```python
from build123d import *

# Parameters (mm, degrees)
F1_DEPTH     = 2.37
F3_DEPTH     = 2.37
F5_DEPTH     = 2.25
F6_DEPTH     = 0.75
F7_SIZE      = 0.5
F8_T4_ANGLE  = 81.836383008
F8_T10_ANGLE = 99.1168662244
F10_DEPTH    = 3.12


# Not quite as in the source:
# - a fillet or chamfer that OpenCascade refuses, or shapes differently, is made with other operations: its cross-section is extruded or revolved along the edge and cut away or added


with BuildPart() as f1:
    # F0 (on Right) → F1 (new body)
    with BuildSketch(Plane.YZ):
        with BuildLine():
            ThreePointArc((-46.5614527995, 89.8296507657), (-59.272592692, 87.6283434753), (-70.5032497848, 81.2808106933))
            Line((-70.5032497848, 81.2808106933), (-46.5614527995, 52.0296507657))
            Line((-46.5614527995, 52.0296507657), (-42.2863249385, 46.8064651858))
            ThreePointArc((-42.2863249385, 46.8064651858), (-37.3697308445, 54.2738686288), (-37.5751261635, 63.2121472344))
            Line((-37.5751261635, 63.2121472344), (-46.5614527995, 89.8296507657))
        make_face()
        with BuildLine():
            Line((-46.5614527995, 52.0296507657), (-70.5032497848, 81.2808106933))
            ThreePointArc((-70.5032497848, 81.2808106933), (-78.9453750126, 71.5263577209), (-83.6157032002, 59.501098232))
            Line((-83.6157032002, 59.501098232), (-59.2995451707, 45.4309163095))
            ThreePointArc((-59.2995451707, 45.4309163095), (-50.5782061954, 43.4628568222), (-42.2863249385, 46.8064651858))
            Line((-42.2863249385, 46.8064651858), (-46.5614527995, 52.0296507657))
        make_face()
    extrude(amount=F1_DEPTH)

    # F2 (on face) → F3 (join)
    with BuildSketch(Plane(origin=(0, 0, 0), x_dir=(0, -1, 0), z_dir=(-1, 0, 0))):
        with BuildLine():
            ThreePointArc((84.0721339402, 59.7652050675), (70.8199402211, 81.6677307982), (46.7301322311, 90.3292793181))
            Line((46.7301322311, 90.3292793181), (46.5614527995, 89.8296507657))
            ThreePointArc((46.5614527995, 89.8296507657), (70.5032497848, 81.2808106933), (83.6157032002, 59.501098232))
            Line((83.6157032002, 59.501098232), (84.0721339402, 59.7652050675))
        make_face()
        with BuildLine():
            ThreePointArc((84.9830454985, 60.2922904452), (71.4533210937, 82.4415710079), (47.0667704776, 91.3264019551))
            Line((47.0667704776, 91.3264019551), (46.7301322311, 90.3292793181))
            ThreePointArc((46.7301322311, 90.3292793181), (70.8199402211, 81.6677307982), (84.0721339402, 59.7652050675))
            Line((84.0721339402, 59.7652050675), (84.9830454985, 60.2922904452))
        make_face()
    extrude(amount=-F3_DEPTH)

    # F4 (on face) → F5 (cut)
    with BuildSketch(Plane.YZ.offset(2.37)):
        with BuildLine():
            ThreePointArc((-73.802497152, 53.8228330154), (-63.8527506222, 73.1554884912), (-42.9348652938, 79.0876969454))
            Line((-42.9348652938, 79.0876969454), (-46.7301322311, 90.3292793181))
            ThreePointArc((-46.7301322311, 90.3292793181), (-70.8199402211, 81.6677307982), (-84.0721339402, 59.7652050675))
            Line((-84.0721339402, 59.7652050675), (-73.802497152, 53.8228330154))
        make_face()
    extrude(amount=-F5_DEPTH, mode=Mode.SUBTRACT)

    # F6 (add): a face of the model
    f6_faces = [f1.faces().sort_by_distance(p)[0] for p in [
        (0, -58.3598378742, 66.4444605195),
    ]]
    extrude(f6_faces, amount=F6_DEPTH)

    # F7
    f7_edges = [f1.edges().sort_by_distance(p)[0] for p in [
        (2.37, -71.453321, 82.441571),
        (2.37, -63.852751, 73.155488),
    ]]
    chamfer(f7_edges, length=F7_SIZE)

    # F8: fillet of radius 0.5 on 2 edges, made by hand


with BuildPart() as f8_tool2:
    # F8_s3 → F8_t4 (revolve)
    with BuildSketch(Plane(origin=(0, -47.9930028953, 1.3558158365), x_dir=(1, 0, 0), z_dir=(0, 0.9996011995, -0.0282390152))):
        with BuildLine():
            ThreePointArc((0.62, -88.9940517429), (0.2664466094, -88.8476051335), (0.12, -88.4940517429))
            Line((0.12, -88.4940517429), (0.12, -88.9940517429))
            Line((0.12, -88.9940517429), (0.62, -88.9940517429))
        make_face()
    revolve(axis=Axis((0.12, -46.5614527995, 52.0296507657), (1, 0, 0)), revolution_arc=F8_T4_ANGLE)

    split(bisect_by=Plane(origin=(0, 4.8196318055, 8.3293115378), x_dir=(1, 0, 0), z_dir=(0, 0.5008338095, 0.8655434681)), keep=Keep.TOP)

    split(bisect_by=Plane(origin=(0, -14.5730530493, -4.9200036596), x_dir=(1, 0, 0), z_dir=(0, -0.947460791, -0.3198719268)), keep=Keep.TOP)


with BuildPart() as f1_1:
    add(f1.part)

    # F8_t1: union F8_tool2
    add(f8_tool2.part)


with BuildPart() as f8_tool8:
    # F8_s9 → F8_t10 (revolve)
    with BuildSketch(Plane(origin=(0, 1.0178886406, 51.0815497106), x_dir=(1, 0, 0), z_dir=(0, -0.0199227826, -0.9998015217))):
        with BuildLine():
            ThreePointArc((0.12, 75.388786783), (0.2664466094, 75.0352333924), (0.62, 74.888786783))
            Line((0.62, 74.888786783), (0.12, 74.888786783))
            Line((0.12, 74.888786783), (0.12, 75.388786783))
        make_face()
    revolve(axis=Axis((0.12, -46.5614527995, 52.0296507657), (-1, 0, 0)), revolution_arc=F8_T10_ANGLE)

    split(bisect_by=Plane(origin=(0, 4.8196318055, 8.3293115378), x_dir=(1, 0, 0), z_dir=(0, 0.5008338095, 0.8655434681)), keep=Keep.TOP)

    split(bisect_by=Plane(origin=(0, -14.5730530493, -4.9200036596), x_dir=(1, 0, 0), z_dir=(0, -0.947460791, -0.3198719268)), keep=Keep.TOP)


with BuildPart() as f1_2:
    add(f1_1.part)

    # F8_t7: union F8_tool8
    add(f8_tool8.part)

    # F9 (on face) → F10 (join)
    with BuildSketch(Plane(origin=(-0.75, 0, 0), x_dir=(0, -1, 0), z_dir=(-1, 0, 0))):
        with BuildLine():
            ThreePointArc((59.2995451707, 45.4309163095), (42.2863249385, 46.8064651858), (37.5751261635, 63.2121472344))
            Line((37.5751261635, 63.2121472344), (33.3301843859, 50.6386277829))
            ThreePointArc((33.3301843859, 50.6386277829), (36.4709835693, 39.7015064172), (47.8131303907, 38.784473833))
            Line((47.8131303907, 38.784473833), (59.2995451707, 45.4309163095))
        make_face()
    extrude(amount=-F10_DEPTH)


solid = f1_2.part
```
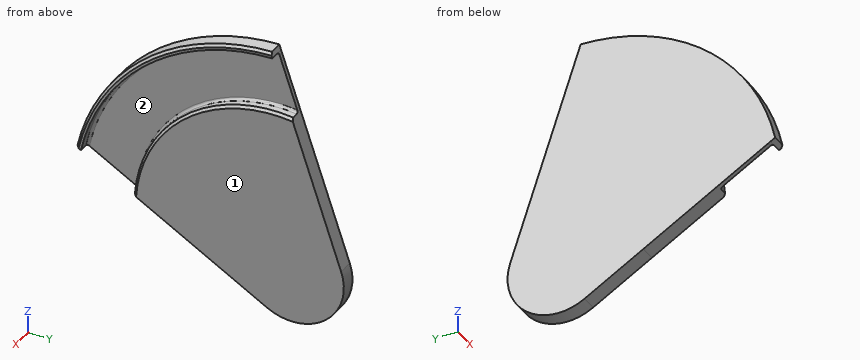
CAD build for the part. Positions are in the model's coordinates, mm. Face numbers are marked on the shaded views. Give positions to 0.01 mm unless a question says otherwise; leave off trailing zeros. Write each loop counter-clockwise with the first axis right and the second up, starting at its lowest first coordinate (ties: lowest second). Pieces come first, ordered by that corner, then holes. Notation, with made-up numbers: M -14.75,63.5 L 17.25,63.5 A10 ccw 17.25,80.5 Z; hole C 48.5,67.25 d11. An arc over 180 degrees is marked long. Return JSON: item names as keys, results as strings. Group by question number.
(1) Mould opens along Z. For the marked faces 1 and 2 say: pulls with the +Z half, pulls with the -Z half, needs draft (parallel to the pull), parting line crosses it, or undercut.
(2) Flat gauge pins, fed straight in: pin 1 Ø1.5 at (x, z) = (1, 65.5) entering from -Y; pin 2 Ø1 at (x, y) = (2, -67.5) entering from -Z; pin 3 Ø1.5 at (x, z) = (1.5, 53) entering from -Y. Where does each tip first touch, or does it go through?
(3) Drill centre lines: L1, parallel to X at y = -56.5, z = 79.5; L2, parallel to Y at x = 0.25, z = 72; L3, parallel to Z at x = 0.75, y = -57. Where is each one in solid material? Low to high. Write a range as [from, to].
(4) Band-saw the part on B-B (z = 48). Give the cut face in (x, y), and give its area (3 significant figures).
(5) Band-saw the part on A-A (x = 1.3). Give the cut face in (y, z), and give its area (3 significant figures).
Entries:
{
 "1": {"face 1": "needs draft", "face 2": "undercut"},
 "2": {"pin 1": "stops at y = -83.75", "pin 2": "stops at z = 49.89", "pin 3": "stops at y = -73.68"},
 "3": {"L1": "x = [-0.75, 0.12]", "L2": "y = [-80.41, -79.05], [-65.41, -40.54]", "L3": "z = [44.1, 77.26], [88.88, 89.92]"},
 "4": {"outline": "M -0.75,-63.74 L 2.37,-63.74 L 2.37,-32.82 L -0.75,-32.82 Z", "area": "96.5 mm^2"},
 "5": {"outline": "M -84.98,60.29 L -84.07,59.77 A38.3 cw -46.73,90.33 L -47.07,91.33 A39.3 ccw Z; M -73.8,53.82 L -47.81,38.78 A10 ccw -33.33,50.64 L -42.93,79.09 A27.3 ccw Z", "area": "1,200 mm^2"}
}
